Here's the drawing with two shaded views (mm, measured from the low corner). I have some questions. Coordinates: 2 decimals unless noted, no trailing zeros. Loops run counter-clockwise (first coordinate to the right, second up) from the corner with the lowest first, then second, coordinate; pieces in that order, holes last. Notation, with made-up numbers: (30.5, 49) - (45.5, 49) arc R25 ccw to (45.5, 64) - close; hole circle Ø10 at (13, 66.25). An arc over 180 degrees is marked (long way). Use a Markdown table: item, result.
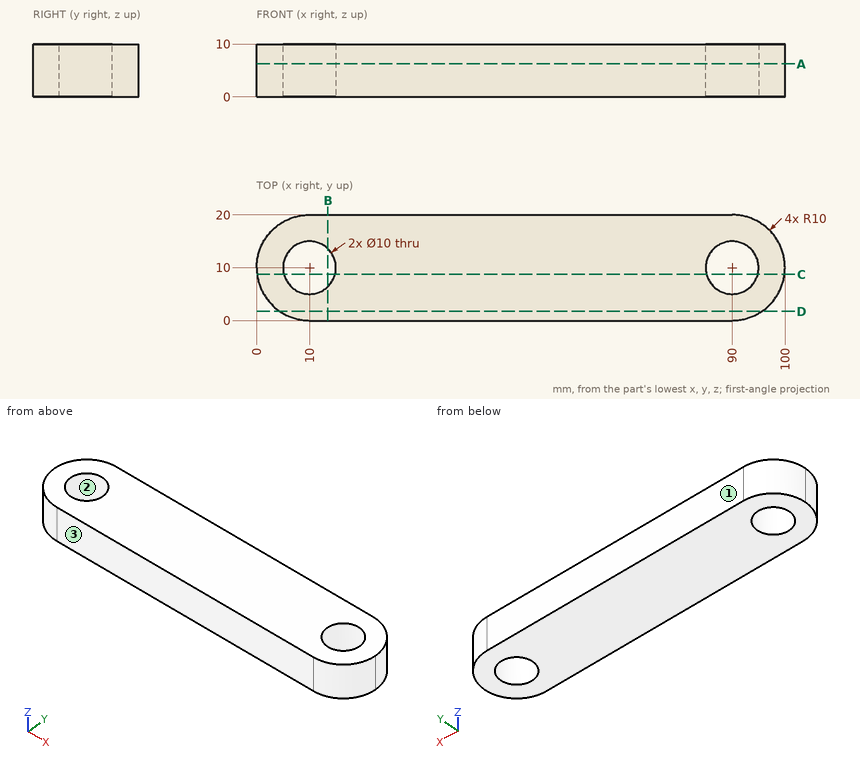
Q1. I want a section at C-C, the plane y = 8.75. Write out the boundary of the cut face in (x, z).
Check values:
| item | result |
|---|---|
| outline | (0.08, 0) - (5.16, 0) - (5.16, 10) - (0.08, 10) - close; (14.84, 0) - (85.16, 0) - (85.16, 10) - (14.84, 10) - close; (94.84, 0) - (99.92, 0) - (99.92, 10) - (94.84, 10) - close |
Q2. I want a section at A-A, the plane z = 6.25. Give the number of separate pieces and of enclosed holes in the cut face, then the cut area to 3 significant figures.
Check values:
| item | result |
|---|---|
| separate pieces | 1 |
| enclosed holes | 2 |
| area | 1,760 mm^2 |
Q3. Please list where these lines run through material, in increasing order: L1, parallel to Y at x = 90, z = 5.5; L2, parallel to X at y = 7.5, z = 2.75; L3, parallel to X at y = 6.5, z = 6.75. Write a range as from..to.
Check values:
| item | result |
|---|---|
| L1 | 0..5, 15..20 |
| L2 | 0.32..5.67, 14.33..85.67, 94.33..99.68 |
| L3 | 0.63..6.43, 13.57..86.43, 93.57..99.37 |
Q4. I want a section at D-D, the plane y = 1.75. Write out the boundary of the cut face in (x, z).
Check values:
| item | result |
|---|---|
| outline | (4.35, 0) - (95.65, 0) - (95.65, 10) - (4.35, 10) - close |
Q5. Will these pins go through, and if not, where does the flat tip stop? P1, Ø6, axis at x = 11, z = 3, coming from the -Y side; P2, Ø6, axis at y = 14.5, z = 8.5, coming from the +X side.
Check values:
| item | result |
|---|---|
| P1 | y = 0 |
| P2 | x = 99.89 |
Q6. I want a section at B-B, the plane x = 13.5. Write out the boundary of the cut face in (y, z).
Check values:
| item | result |
|---|---|
| outline | (0, 0) - (6.43, 0) - (6.43, 10) - (0, 10) - close; (13.57, 0) - (20, 0) - (20, 10) - (13.57, 10) - close |
Q7. If we mould it in two halves opening along Y, with no side actions, what happens to the marked faces 1, 2 and 3? For each: pulls with the +Y half, pulls with the -Y half, needs draft (parallel to the pull), parting line crosses it, or undercut.
Check values:
| item | result |
|---|---|
| face 1 | pulls with the +Y half |
| face 2 | undercut |
| face 3 | pulls with the -Y half |
